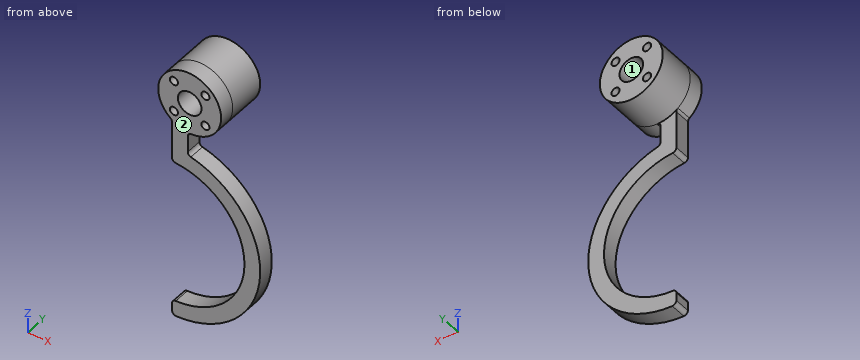
from build123d import *

# Parameters (mm, degrees)
SKETCH1_R           = 2.075
SKETCH1_R_2         = 6.003208263
BOSS_EXTRUDE2_DEPTH = 8
FILLET1_R           = 2
SKETCH2_R           = 16
SKETCH2_R_2         = 2.075
SKETCH2_R_3         = 6.003208263
SKETCH2_R_4         = 2.059067384
BOSS_EXTRUDE3_DEPTH = 19


with BuildPart() as part:
    # Sketch1 → Boss-Extrude2 (new body)
    with BuildSketch(Plane(origin=(0, 0, 0), x_dir=(1, 0, 0), z_dir=(0, 1, 0))):
        with BuildLine():
            Line((0, 44.83), (0, 36.83))
            ThreePointArc((0, 36.83), (36.83, 0), (0, -36.83))
            Line((0, -36.83), (0, -46.83))
            Line((0, -46.83), (0, -58.83))
            ThreePointArc((0, -58.83), (14.116701064, -87.229775601), (8, -56.110417137))
            Line((8, -56.110417137), (8, -44.110417137))
            ThreePointArc((8, -44.110417137), (44.649741882, 4.016148637), (0, 44.83))
        make_face()
        with Locations(Location((0.96696537, -64.081170969, 0), (0, 0, 270))):
            Circle(SKETCH1_R, mode=Mode.SUBTRACT)
        with Locations(Location((16.96696537, -64.081170969, 0), (0, 0, 270))):
            Circle(SKETCH1_R, mode=Mode.SUBTRACT)
        with Locations(Location((16.96696537, -80.081170969, 0), (0, 0, 270))):
            Circle(SKETCH1_R, mode=Mode.SUBTRACT)
        with Locations(Location((0.96696537, -80.081170969, 0), (0, 0, 270))):
            Circle(SKETCH1_R, mode=Mode.SUBTRACT)
        with Locations(Location((8.96696537, -72.081170969, 0), (0, 0, 270))):
            Circle(SKETCH1_R_2, mode=Mode.SUBTRACT)
    extrude(amount=BOSS_EXTRUDE2_DEPTH)

    # Fillet1
    fillet1_edges = [part.edges().sort_by_distance(p)[0] for p in [
        (0, 4, 58.83),
        (0, 4, 36.83),
        (0, 4, -36.83),
        (0, 4, -44.83),
        (8, 4, 44.110417137),
        (8, 4, 56.110417137),
    ]]
    fillet(fillet1_edges, radius=FILLET1_R)

    # Sketch2 → Boss-Extrude3 (add)
    with BuildSketch(Plane(origin=(0, 8, 0), x_dir=(1, 0, 0), z_dir=(0, 1, 0))):
        with Locations(Location((8.96696537, -72.081170969, 0), (0, 0, 86.709940875))):
            Circle(SKETCH2_R)
        with Locations(Location((0.96696537, -64.081170969, 0), (0, 0, 270))):
            Circle(SKETCH2_R_2, mode=Mode.SUBTRACT)
        with Locations(Location((8.96696537, -72.081170969, 0), (0, 0, 270))):
            Circle(SKETCH2_R_3, mode=Mode.SUBTRACT)
        with Locations(Location((16.96696537, -64.081170969, 0), (0, 0, 270))):
            Circle(SKETCH2_R_2, mode=Mode.SUBTRACT)
        with Locations(Location((16.96696537, -80.081170969, 0), (0, 0, 270))):
            Circle(SKETCH2_R_4, mode=Mode.SUBTRACT)
        with Locations(Location((0.96696537, -80.081170969, 0), (0, 0, 270))):
            Circle(SKETCH2_R_2, mode=Mode.SUBTRACT)
    extrude(amount=BOSS_EXTRUDE3_DEPTH)


solid = part.part
Could you check a few things on this model? Use its own coordinates, in mm. Face numbers are marked on the shaded views. Give positions to 0.01 mm unless a question says otherwise; leave off trailing zeros. Write each loop counter-clockwise with the first axis right and the second up, starting at its lowest first coordinate (ties: lowest second). Pieces come first, ordered by that corner, then holes. Notation, with made-up numbers: (-1, -21.5) -> (8, -21.5) arc R19 cw to (8, -2.5) -> close; hole circle Ø8 at (-8, 26.25). An arc over 180 degrees is marked (long way). Answer as CSV lines item,"result". Start each with the question number.
(1) If we section it at B-B, the plane y = 3.5: Write out the boundary of the cut face in (x, z) (3 decimals).
(2) If we section it at C-C, the plane z = 0: Write out the boundary of the cut face in (x, y).
(3) If we section it at D-D, the plane y = 19.75: Write out the boundary of the cut face in (x, z) (3 decimals).
(4) Please list where these lines run through material, in increasing order: line 1 (Z direction, x = 9.5, y = 24.5); line 2 (Z direction, x = 15.5, y = 5.75); line 3 (Z direction, x = 1, y = 15.75).
(5) I'm going to push flat-ended pins straight in: pin 1 Ø23 at (x, z) = (24.5, 32.5) entering from +Y; pin 2 Ø2.5 at (y, z) = (5.5, 48.5) entering from +X; pin 3 Ø2 at (y, z) = (4.5, -40.5) entering from -X. Where does each tip first touch, or does it pass through?
(6) If we section it at A-A, the plane x = 22.5: Write out the boundary of the cut face in (y, z), and give its area (3 significant figures).
(7) If we mould it in two halves opening along Z, with no side actions, what happens to the marked faces 1 and 2? For each: +Z half, -Z half, draft (parallel to the pull), parting line (faces both ways), or undercut.
Answer list:
1,outline,"(-0.781, 59.394) arc R2 cw to (0, 57.808) -> (0, 38.778) arc R2 ccw to (1.897, 36.781) arc R36.83 cw to (1.897, -36.781) arc R2 ccw to (0, -38.778) -> (0, -42.783) arc R2 ccw to (2.093, -44.781) arc R44.83 ccw to (9.573, 43.796) arc R2 cw to (8, 45.75) -> (8, 54.111) arc R2 cw to (9.885, 56.108) arc R16 ccw (long way) to start; hole circle Ø4.15 at (0.967, 64.081); hole circle Ø4.15 at (0.967, 80.081); hole circle Ø12.006 at (8.967, 72.081); hole circle Ø4.15 at (16.967, 64.081); hole circle Ø4.15 at (16.967, 80.081)"
2,outline,"(36.83, 0) -> (44.83, 0) -> (44.83, 8) -> (36.83, 8) -> close"
3,outline,"circle Ø32 at (8.967, 72.081); hole circle Ø4.15 at (0.967, 64.081); hole circle Ø4.15 at (0.967, 80.081); hole circle Ø12.006 at (8.967, 72.081); hole circle Ø4.15 at (16.967, 64.081); hole circle Ø4.118 at (16.967, 80.081)"
4,line 1,"56.09 to 66.1, 78.06 to 88.07"
4,line 2,"-42.07 to -33.41, 33.41 to 42.07, 57.48 to 62.61, 65.55 to 78.61, 81.55 to 86.69"
4,line 3,"58.21 to 62.01, 66.16 to 78.01, 82.16 to 85.96"
5,pin 1,"y = 8"
5,pin 2,"x = 8"
5,pin 3,"x = 0"
6,outline,"(0, -38.77) -> (8, -38.77) -> (8, -29.16) -> (0, -29.16) -> close; (0, 29.16) -> (8, 29.16) -> (8, 38.77) -> (0, 38.77) -> close; (0, 63.55) -> (27, 63.55) -> (27, 80.62) -> (0, 80.62) -> close"
6,area,"615 mm^2"
7,face 1,"undercut"
7,face 2,"draft"
